Model file for the job. Use its own axes, mm. Round coordinates to 2 decimals unless told otherwise and drop trailing zeros. Order: outer loops, then holes, each group sorted by start corner. A loop starts at its lowest first (then second) coordinate and runs counter-clockwise, first axis right, second up. Notation, with made-up numbers: (61.25, -37.75) -> (103.25, -37.75) arc R12 ccw to (103.25, -19.75) -> close; hole circle Ø10 at (56.25, -31). An arc over 180 degrees is marked (long way). Answer as CSV lines item,"result".
```python
from build123d import *

# Parameters (mm, degrees)
F0_W         = 140
F0_H         = 70
F1_DEPTH     = 7
F2_R         = 10
F3_R         = 0.7
F4_R         = 3
F6_DEPTH     = 1
F7_R         = 2
F8_T1_DEPTH  = 8
F8_T3_DEPTH  = 8
F8_T6_ANGLE  = 90
F8_T8_ANGLE  = 90
F8_T10_ANGLE = 90
F8_T12_ANGLE = 90
F9_DEPTH     = 0.5
F10_R        = 1.5
F11_DEPTH    = 0.1


# Not quite as in the source:
# - a fillet or chamfer that OpenCascade refuses, or shapes differently, is made with other operations: its cross-section is extruded or revolved along the edge and cut away or added


with BuildPart() as f1:
    # F0 (on Top) → F1 (new body)
    with BuildSketch(Plane.XY):
        with Locations((18.6064650118, 35)):
            Rectangle(F0_W, F0_H)
    extrude(amount=F1_DEPTH)

    # F2
    f2_edges = [f1.edges().sort_by_distance(p)[0] for p in [
        (88.606465, 70, 3.5),
        (88.606465, 0, 3.5),
        (-51.393535, 0, 3.5),
        (-51.393535, 70, 3.5),
    ]]
    fillet(f2_edges, radius=F2_R)

    # F3
    f3_edges = [f1.edges().sort_by_distance(p)[0] for p in [
        (18.606465, 0, 7),
        (88.606465, 35, 7),
        (85.677533, 2.928932, 7),
        (85.677533, 67.071068, 7),
        (18.606465, 70, 7),
        (-48.464603, 2.928932, 7),
        (-48.464603, 67.071068, 7),
        (-51.393535, 35, 7),
    ]]
    fillet(f3_edges, radius=F3_R)

    # F4
    f4_edges = [f1.edges().sort_by_distance(p)[0] for p in [
        (18.606465, 0, 0),
        (88.606465, 35, 0),
        (85.677533, 2.928932, 0),
        (85.677533, 67.071068, 0),
        (18.606465, 70, 0),
        (-48.464603, 2.928932, 0),
        (-48.464603, 67.071068, 0),
        (-51.393535, 35, 0),
    ]]
    fillet(f4_edges, radius=F4_R)

    # F5 (on face) → F6 (join)
    with BuildSketch(Plane(origin=(0, 0, 0), x_dir=(1, 0, 0), z_dir=(0, 0, -1))):
        Polygon((78.6064650118, -41), (78.6064650118, -35), (78.6064650118, -29), (66.6064650118, -29), (66.6064650118, -41), align=None)
    extrude(amount=F6_DEPTH)

    # F7
    f7_edges = [f1.edges().sort_by_distance(p)[0] for p in [
        (66.606465, 41, -0.5),
        (66.606465, 29, -0.5),
        (78.606465, 29, -0.5),
        (78.606465, 41, -0.5),
    ]]
    fillet(f7_edges, radius=F7_R)

    # F8: fillet of radius 2 on 1 edges, made by hand

    # F8_s2 → F8_t1 (cut)
    with BuildSketch(Plane.YZ.offset(68.6064650118)):
        with BuildLine():
            ThreePointArc((41, 0), (40.2679491924, -0.7320508076), (39.2679491924, -1))
            Line((39.2679491924, -1), (41, -1))
            Line((41, -1), (41, 0))
        make_face()
        with BuildLine():
            ThreePointArc((29, 0), (29.7320508076, -0.7320508076), (30.7320508076, -1))
            Line((30.7320508076, -1), (29, -1))
            Line((29, -1), (29, 0))
        make_face()
    extrude(amount=F8_T1_DEPTH, mode=Mode.SUBTRACT)

    # F8_s4 → F8_t3 (cut)
    with BuildSketch(Plane.XZ.offset(-39)):
        with BuildLine():
            ThreePointArc((78.6064650118, 0), (77.8744142043, -0.7320508076), (76.8744142043, -1))
            Line((76.8744142043, -1), (78.6064650118, -1))
            Line((78.6064650118, -1), (78.6064650118, 0))
        make_face()
        with BuildLine():
            ThreePointArc((66.6064650118, 0), (67.3385158194, -0.7320508076), (68.3385158194, -1))
            Line((68.3385158194, -1), (66.6064650118, -1))
            Line((66.6064650118, -1), (66.6064650118, 0))
        make_face()
    extrude(amount=F8_T3_DEPTH, mode=Mode.SUBTRACT)

    # F8_s5 → F8_t6 (revolve, cut)
    with BuildSketch(Plane.YZ.offset(68.6064650118)):
        with BuildLine():
            ThreePointArc((41, 0), (40.2679491924, -0.7320508076), (39.2679491924, -1))
            Line((39.2679491924, -1), (41, -1))
            Line((41, -1), (41, 0))
        make_face()
    revolve(axis=Axis((68.6064650118, 39, -1), (0, 0, 1)), revolution_arc=F8_T6_ANGLE, mode=Mode.SUBTRACT)

    # F8_s7 → F8_t8 (revolve, cut)
    with BuildSketch(Plane.YZ.offset(76.6064650118)):
        with BuildLine():
            ThreePointArc((41, 0), (40.2679491924, -0.7320508076), (39.2679491924, -1))
            Line((39.2679491924, -1), (41, -1))
            Line((41, -1), (41, 0))
        make_face()
    revolve(axis=Axis((76.6064650118, 39, -1), (0, 0, -1)), revolution_arc=F8_T8_ANGLE, mode=Mode.SUBTRACT)

    # F8_s9 → F8_t10 (revolve, cut)
    with BuildSketch(Plane.YZ.offset(76.6064650118)):
        with BuildLine():
            ThreePointArc((29, 0), (29.7320508076, -0.7320508076), (30.7320508076, -1))
            Line((30.7320508076, -1), (29, -1))
            Line((29, -1), (29, 0))
        make_face()
    revolve(axis=Axis((76.6064650118, 31, -1), (0, 0, 1)), revolution_arc=F8_T10_ANGLE, mode=Mode.SUBTRACT)

    # F8_s11 → F8_t12 (revolve, cut)
    with BuildSketch(Plane.XZ.offset(-31)):
        with BuildLine():
            ThreePointArc((66.6064650118, 0), (67.3385158194, -0.7320508076), (68.3385158194, -1))
            Line((68.3385158194, -1), (66.6064650118, -1))
            Line((66.6064650118, -1), (66.6064650118, 0))
        make_face()
    revolve(axis=Axis((68.6064650118, 31, -1), (0, 0, 1)), revolution_arc=F8_T12_ANGLE, mode=Mode.SUBTRACT)

    # F9 (cut): faces of the model
    f9_faces = [f1.faces().sort_by_distance(p)[0] for p in [
        (72.6064650118, 35, -1),
        (17.7021104435, 35, 0),
    ]]
    extrude(f9_faces, amount=F9_DEPTH, mode=Mode.SUBTRACT)

    # F10 (on face) → F11 (cut)
    with BuildSketch(Plane(origin=(0, 0, -1), x_dir=(1, 0, 0), z_dir=(0, 0, -1))):
        with Locations((72.6282298565, -35)):
            Circle(F10_R)
    extrude(amount=-F11_DEPTH, mode=Mode.SUBTRACT)


solid = f1.part
```
Q1. Flat gauge pins, fed straight in: pin 1 (0.9 mm diameter, centred on x = 72.5, y = 35, fed in from -Z); pin 2 (2 mm diameter, centred on y = 30, z = 1, fed in from +X); pin 3 (19 mm diameter, centred on x = -4, y = 35.5, fed in from -Z). Where does each tip first touch, or does it go through?
Checks:
pin 1,"z = -0.9"
pin 2,"x = 88.43"
pin 3,"z = 0"
Q2. Mould opens along Y. For faces 1 (the flat face through (73, 35, -0.9)), 2 (the cylindrical face through (85.6, 2.85, 4.67)), 3 (the cylindrical face through (17.77, 69.1, 0.86)) say: +Y half, -Y half, draft (parallel to the pull), parting line (faces both ways), or undercut.
Checks:
face 1,"undercut"
face 2,"-Y half"
face 3,"+Y half"
Q3. Saw through at C-C (y = 35). Write the cut outline in (x, z), plus the area to 3 significant figures.
Checks:
outline,"(-51.39, 3) arc R3 ccw to (-48.39, 0) -> (66.61, 0) arc R2 ccw to (68.34, -1) -> (71.13, -1) -> (71.13, -0.9) -> (74.13, -0.9) -> (74.13, -1) -> (76.87, -1) arc R2 ccw to (78.61, 0) -> (85.61, 0) arc R3 ccw to (88.61, 3) -> (88.61, 6.3) arc R0.7 ccw to (87.91, 7) -> (-50.69, 7) arc R0.7 ccw to (-51.39, 6.3) -> close"
area,"987 mm²"
Q4. Saw through at A-A (x = -9.5). Write the cut outline in (y, z).
Checks:
outline,"(0, 3) arc R3 ccw to (3, 0) -> (67, 0) arc R3 ccw to (70, 3) -> (70, 6.3) arc R0.7 ccw to (69.3, 7) -> (0.7, 7) arc R0.7 ccw to (0, 6.3) -> close"
Q5. Wall check: L1, parallel to Z at x = 14, y = 63.5; L2, parallel to Y at x = -42, z = 0.5; L3, parallel to Y at x = -23, z = 2. Give the ranges that are in metal, low to high. Write a range as [from, to].
Checks:
L1,"[0, 7]"
L2,"[1.36, 68.64]"
L3,"[0.17, 69.83]"
Q6. Saw through at B-B (y = 47). Write the cut outline in (x, z).
Checks:
outline,"(-51.39, 3) arc R3 ccw to (-48.39, 0) -> (85.61, 0) arc R3 ccw to (88.61, 3) -> (88.61, 6.3) arc R0.7 ccw to (87.91, 7) -> (-50.69, 7) arc R0.7 ccw to (-51.39, 6.3) -> close"
